```python
from build123d import *

# Parameters (mm, degrees)
SKETCH1_W                            = 140
SKETCH1_H                            = 90
BOSS_EXTRUDE1_DEPTH                  = 6
FILLET1_R                            = 3
SKETCH2_W                            = 100
SKETCH2_H                            = 50
CUT_EXTRUDE1_DEPTH                   = 10
FILLET2_R                            = 3
F_2_9_2_9_DIAMETER_HOLE1_D           = 2.9
F_2_9_2_9_DIAMETER_HOLE1_DEPTH       = 15
F_2_9_2_9_DIAMETER_HOLE1_CSINK_D     = 2.95
F_2_9_2_9_DIAMETER_HOLE1_CSINK_ANGLE = 90
F_2_9_2_9_DIAMETER_HOLE1_TIP         = 0.871247898
F_2_9_2_9_DIAMETER_HOLE2_D           = 2.9
F_2_9_2_9_DIAMETER_HOLE2_DEPTH       = 15
F_2_9_2_9_DIAMETER_HOLE2_CSINK_D     = 2.95
F_2_9_2_9_DIAMETER_HOLE2_CSINK_ANGLE = 90
F_2_9_2_9_DIAMETER_HOLE2_TIP         = 0.871247898
SKETCH7_R                            = 4.25
CUT_EXTRUDE2_DEPTH                   = 3
F_4_3_4_3_DIAMETER_HOLE1_D           = 4.3
F_4_3_4_3_DIAMETER_HOLE1_DEPTH       = 15
F_4_3_4_3_DIAMETER_HOLE1_CSINK_D     = 4.35
F_4_3_4_3_DIAMETER_HOLE1_CSINK_ANGLE = 90
F_4_3_4_3_DIAMETER_HOLE1_TIP         = 1.291850331


with BuildPart() as part:
    # Sketch1 → Boss-Extrude1 (new body)
    with BuildSketch(Plane(origin=(0, 0, 0), x_dir=(1, 0, 0), z_dir=(0, 1, 0))):
        Rectangle(SKETCH1_W, SKETCH1_H)
    extrude(amount=BOSS_EXTRUDE1_DEPTH)

    # Fillet1
    fillet1_edges = [part.edges().sort_by_distance(p)[0] for p in [
        (70, 3, 45),
        (-70, 3, 45),
        (-70, 3, -45),
        (70, 3, -45),
    ]]
    fillet(fillet1_edges, radius=FILLET1_R)

    # Sketch2 → Cut-Extrude1 (cut)
    with BuildSketch(Plane(origin=(0, 6, 0), x_dir=(1, 0, 0), z_dir=(0, 1, 0))):
        Rectangle(SKETCH2_W, SKETCH2_H)
    extrude(amount=-CUT_EXTRUDE1_DEPTH, mode=Mode.SUBTRACT)

    # Fillet2
    fillet2_edges = [part.edges().sort_by_distance(p)[0] for p in [
        (50, 3, -25),
        (50, 3, 25),
        (-50, 3, 25),
        (-50, 3, -25),
    ]]
    fillet(fillet2_edges, radius=FILLET2_R)

    # Ø2.9 (2.9) Diameter Hole1
    with Locations(Plane(origin=(0, 6, 0), x_dir=(1, 0, 0), z_dir=(0, 1, 0))):
        with Locations((0, 0), (-52.5, 16.5), (-52.5, 8.5), (-52.5, -8.5), (-52.5, -16.5), (52.5, 16.5), (52.5, 8.5), (52.5, -8.5), (52.5, -16.5)):
            CounterSinkHole(F_2_9_2_9_DIAMETER_HOLE1_D / 2, F_2_9_2_9_DIAMETER_HOLE1_CSINK_D / 2, depth=F_2_9_2_9_DIAMETER_HOLE1_DEPTH, counter_sink_angle=F_2_9_2_9_DIAMETER_HOLE1_CSINK_ANGLE)
            with Locations((0, 0, -(F_2_9_2_9_DIAMETER_HOLE1_DEPTH + F_2_9_2_9_DIAMETER_HOLE1_TIP / 2))):  # 118° drill point
                Cone(0, F_2_9_2_9_DIAMETER_HOLE1_D / 2, F_2_9_2_9_DIAMETER_HOLE1_TIP, mode=Mode.SUBTRACT)

    # Ø2.9 (2.9) Diameter Hole2
    with Locations(Plane(origin=(0, 6, 0), x_dir=(1, 0, 0), z_dir=(0, 1, 0))):
        with Locations((0, 0), (30, -30), (-30, 30), (-30, -30), (30, 30)):
            CounterSinkHole(F_2_9_2_9_DIAMETER_HOLE2_D / 2, F_2_9_2_9_DIAMETER_HOLE2_CSINK_D / 2, depth=F_2_9_2_9_DIAMETER_HOLE2_DEPTH, counter_sink_angle=F_2_9_2_9_DIAMETER_HOLE2_CSINK_ANGLE)
            with Locations((0, 0, -(F_2_9_2_9_DIAMETER_HOLE2_DEPTH + F_2_9_2_9_DIAMETER_HOLE2_TIP / 2))):  # 118° drill point
                Cone(0, F_2_9_2_9_DIAMETER_HOLE2_D / 2, F_2_9_2_9_DIAMETER_HOLE2_TIP, mode=Mode.SUBTRACT)

    # Sketch7 → Cut-Extrude2 (cut)
    with BuildSketch(Plane(origin=(0, 6, 0), x_dir=(1, 0, 0), z_dir=(0, 1, 0))):
        with Locations(Location((-30, 30, 0), (0, 0, 270))):
            Circle(SKETCH7_R)
        with Locations(Location((30, 30, 0), (0, 0, 270))):
            Circle(SKETCH7_R)
        with Locations(Location((30, -30, 0), (0, 0, 270))):
            Circle(SKETCH7_R)
        with Locations(Location((-30, -30, 0), (0, 0, 270))):
            Circle(SKETCH7_R)
    extrude(amount=-CUT_EXTRUDE2_DEPTH, mode=Mode.SUBTRACT)

    # Ø4.3 (4.3) Diameter Hole1
    with Locations(Plane(origin=(0, 6, 0), x_dir=(1, 0, 0), z_dir=(0, 1, 0))):
        with Locations((0, 0), (64, -39), (-64, 39), (-64, -39), (64, 39)):
            CounterSinkHole(F_4_3_4_3_DIAMETER_HOLE1_D / 2, F_4_3_4_3_DIAMETER_HOLE1_CSINK_D / 2, depth=F_4_3_4_3_DIAMETER_HOLE1_DEPTH, counter_sink_angle=F_4_3_4_3_DIAMETER_HOLE1_CSINK_ANGLE)
            with Locations((0, 0, -(F_4_3_4_3_DIAMETER_HOLE1_DEPTH + F_4_3_4_3_DIAMETER_HOLE1_TIP / 2))):  # 118° drill point
                Cone(0, F_4_3_4_3_DIAMETER_HOLE1_D / 2, F_4_3_4_3_DIAMETER_HOLE1_TIP, mode=Mode.SUBTRACT)


solid = part.part
```
The model under review builds one solid part; all positions refer to its coordinate system, in mm. A direction names the side the tool comes from. Coordinates: 2 decimals unless noted, no trailing zeros. Write each loop counter-clockwise with the first axis right and the second up, starting at its lowest first coordinate (ties: lowest second). Pieces come first, ordered by that corner, then holes. Notation, with made-up numbers: (34, 41) - (80, 41) arc R32 ccw to (80, 75) - close; hole circle Ø11 at (80.5, 63). An arc over 180 degrees is marked (long way). Write item = value, one per line.
(1) Consider section D-D, the plane x = 30. Give the boundary of the cut face in (y, z), then the cut area to 3 significant figures.
Result sheet:
outline = (0, -45) - (6, -45) - (6, -34.25) - (3, -34.25) - (3, -31.45) - (0, -31.45) - close; (0, -28.55) - (3, -28.55) - (3, -25.75) - (6, -25.75) - (6, -25) - (0, -25) - close; (0, 25) - (6, 25) - (6, 25.75) - (3, 25.75) - (3, 28.55) - (0, 28.55) - close; (0, 31.45) - (3, 31.45) - (3, 34.25) - (6, 34.25) - (6, 45) - (0, 45) - close
area = 172 mm^2
(2) For line 1 (Z direction, x = 52.5, y = 3.2); line 2 (X direction, y = 4.15, z = -8.5); line 3 (Z direction, x = 29.5, y = 3.3), list the stretches that pass through material, from the lowest coordinate up. Write a range as [from, to].
Result sheet:
line_1 = [-45, -17.95], [-15.05, -9.95], [-7.05, 7.05], [9.95, 15.05], [17.95, 45]
line_2 = [-70, -53.95], [-51.05, -50], [50, 51.05], [53.95, 70]
line_3 = [-45, -34.22], [-25.78, -25], [25, 25.78], [34.22, 45]
(3) Machinability: for faces 1 (the face through (-1, 3, 25)), 2 (the face through (30, 3, 32)), 3 (the face through (-1, 3, 45)), which of the approach directions +Z, -Z, +X, -X, +Y, -Y give a long, thin tool a straight path to every point of the face, cutting with its end or side? Answer none if there is none.
Result sheet:
face_1 = +Y, -Y
face_2 = +Y
face_3 = +Z, +X, -X, +Y, -Y
(4) Consider section A-A, the plane x = -52.5. Give the boundary of the cut face in (y, z) (3 decimals).
Result sheet:
outline = (0, -45) - (6, -45) - (6, -17.975) - (5.975, -17.95) - (0, -17.95) - close; (0, -15.05) - (5.975, -15.05) - (6, -15.025) - (6, -9.975) - (5.975, -9.95) - (0, -9.95) - close; (0, -7.05) - (5.975, -7.05) - (6, -7.025) - (6, 7.025) - (5.975, 7.05) - (0, 7.05) - close; (0, 9.95) - (5.975, 9.95) - (6, 9.975) - (6, 15.025) - (5.975, 15.05) - (0, 15.05) - close; (0, 17.95) - (5.975, 17.95) - (6, 17.975) - (6, 45) - (0, 45) - close
(5) Consider section C-C, the plane y = 4.3. State how many separate pieces and enclosed holes the cut face has, then the cut area to 3 significant figures.
Result sheet:
separate_pieces = 1
enclosed_holes = 17
area = 7,260 mm^2
(6) Mouldability with a two-part tool opening along X and no side actions: class faces 4 (the face through (69.14, 3.04, -44.1)), 5 (the face through (-50, 3, 0)), 6 (the face through (-69.14, 3.04, -44.1)) as pulls with the +X half, pulls with the -X half, needs draft (parallel to the pull), parting line crosses it, or undercut.
Result sheet:
face_4 = pulls with the +X half
face_5 = undercut
face_6 = pulls with the -X half
(7) Consider section B-B, the plane z = -30. Give the boundary of the cut face in (x, y), then the cut area to 3 significant figures.
Result sheet:
outline = (-70, 0) - (-31.45, 0) - (-31.45, 3) - (-34.25, 3) - (-34.25, 6) - (-70, 6) - close; (-28.55, 0) - (28.55, 0) - (28.55, 3) - (25.75, 3) - (25.75, 6) - (-25.75, 6) - (-25.75, 3) - (-28.55, 3) - close; (31.45, 0) - (70, 0) - (70, 6) - (34.25, 6) - (34.25, 3) - (31.45, 3) - close
area = 772 mm^2
(8) For P1, Ø5, axis at x = 30, z = 30, coming from the +Y side, flat-tipped, find the tip position at first contact; note if it passes through.
Result sheet:
P1 = 3
